Autodesk Inventor part; units mm, degrees
ref_plane "YZ Plane" through (0, 0, 0) normal (1, 0, 0) x (0, 1, 0)
ref_plane "XZ Plane" through (0, 0, 0) normal (0, 1, 0) x (-1, 0, 0)
ref_plane "XY Plane" through (0, 0, 0) normal (0, 0, 1) x (1, 0, 0)
sketch "スケッチ1" plane through (0, 0, 0) normal (0, 0, 1) x (1, 0, 0)
  line L0 (67.5, 17.5) -> (-67.5, 17.5) construction
  line L1 (-67.5, 17.5) -> (-67.5, -17.5) construction
  line L2 (-67.5, -17.5) -> (67.5, -17.5) construction
  line L3 (67.5, -17.5) -> (67.5, 17.5) construction
  line L4 (67.5, 17.5) -> (-67.5, -17.5) construction
  line L5 (-67.5, 17.5) -> (67.5, -17.5) construction
  circle A0 centre (-60, 35) radius 1.6
  circle A1 centre (-70, 35) radius 1.6
  line L6 (-77.5, 27.5) -> (-53, 27.5)
  line L7 (-53, 27.5) -> (-53, 42.5)
  line L8 (-53, 42.5) -> (-80, 42.5) construction
  line L9 (-77.5, 27.5) -> (-77.5, -27.5)
  line L10 (-77.5, -27.5) -> (-50, -27.5)
  circle A2 centre (-60, -35) radius 1.6
  circle A3 centre (-70, -35) radius 1.6
  circle A4 centre (-80, -35) radius 1.6
  line L11 (124.2308, -31.7536) -> (484.5935, -392.1164)
  line L12 (484.5935, -392.1164) -> (488.7129, -553.575)
  line L13 (-80, 21.2868) -> (-468.838, -367.5512) construction
  line L14 (-468.838, -367.5512) -> (-479.4446, -356.9446)
  line L15 (-479.4446, -356.9446) -> (-90.6066, 31.8934) construction
  line L16 (-90.6066, 31.8934) -> (-80, 21.2868) construction
  line L17 (-80, 42.5) -> (-80, 5.3052) construction
  circle A5 centre (-92.3744, 19.519) radius 1.6
  circle A6 centre (-102.981, 8.9124) radius 1.6
  circle A7 centre (-113.5876, -1.6942) radius 1.6
  line L18 (-92.3744, 19.519) -> (-113.5876, -1.6942) construction
  circle A8 centre (-433.75, -321.8566) radius 1.6
  circle A9 centre (-421.9492, -310.0558) radius 1.6
  line L19 (-388.4374, -772.2067) -> (-358.1265, -754.7067) construction
  line L20 (-358.1265, -754.7067) -> (-425.6265, -637.7933) construction
  line L21 (-455.9374, -655.2933) -> (-358.1265, -754.7067) construction
  line L22 (-388.4374, -772.2067) -> (-425.6265, -637.7933) construction
  line L23 (-455.9374, -655.2933) -> (-388.4374, -772.2067) construction
  line L24 (-425.6265, -637.7933) -> (-455.9374, -655.2933) construction
  line L25 (455.9374, -655.2933) -> (425.6265, -637.7933) construction
  line L26 (425.6265, -637.7933) -> (358.1265, -754.7067) construction
  line L27 (388.4374, -772.2067) -> (425.6265, -637.7933) construction
  line L28 (455.9374, -655.2933) -> (358.1265, -754.7067) construction
  line L29 (388.4374, -772.2067) -> (455.9374, -655.2933) construction
  line L30 (358.1265, -754.7067) -> (388.4374, -772.2067) construction
  line L31 (0, 0) -> (0, -263.4473) construction
  line L32 (67.5, 17.5) -> (67.5, -17.5) construction
  circle A10 centre (60, 35) radius 1.6
  circle A11 centre (70, 35) radius 1.6
  line L33 (77.5, 27.5) -> (53, 27.5)
  line L34 (53, 27.5) -> (53, 42.5)
  line L35 (53, 42.5) -> (80, 42.5)
  line L36 (77.5, 27.5) -> (77.5, -27.5)
  line L37 (77.5, -27.5) -> (50, -27.5)
  line L38 (50, -27.5) -> (72.3664, -42.5)
  line L39 (72.3664, -42.5) -> (99.3664, -42.5)
  circle A12 centre (60, -35) radius 1.6
  circle A13 centre (70, -35) radius 1.6
  circle A14 centre (80, -35) radius 1.6
  line L40 (80, 42.5) -> (80, 5.3052) construction
  line L41 (-483.838, -367.5512) -> (-468.838, -367.5512)
  line L42 (-468.838, -367.5512) -> (-468.838, -648.3077)
  line L43 (-468.838, -648.3077) -> (-483.838, -648.3077)
  line L44 (-483.838, -648.3077) -> (-483.838, -367.5512)
  line L45 (-283.2277, -604.4352) -> (-262.2277, -640.8083) construction
  line L46 (345.2492, -497.0108) -> (305.7786, -565.3759) construction
  line L47 (265.1134, -631.6538) -> (-234.8866, -631.6538) construction
  line L48 (-234.8866, -631.6538) -> (-234.8866, -1131.6538) construction
  line L49 (-234.8866, -1131.6538) -> (265.1134, -1131.6538) construction
  line L50 (265.1134, -1131.6538) -> (265.1134, -631.6538) construction
  line L51 (265.1134, -631.6538) -> (-234.8866, -1131.6538) construction
  line L52 (-234.8866, -631.6538) -> (265.1134, -1131.6538) construction
  line L53 (-12.841, -157.5) -> (15.1134, -157.5) construction
  circle A15 centre (1.1362, -409.4569) radius 212.5 construction
  line L54 (501.1362, 53.616) -> (-498.8638, 53.616) construction
  line L55 (-498.8638, 53.616) -> (-498.8638, -946.384) construction
  line L56 (-498.8638, -946.384) -> (501.1362, -946.384) construction
  line L57 (501.1362, -946.384) -> (501.1362, 53.616) construction
  line L58 (501.1362, 53.616) -> (-498.8638, -946.384) construction
  line L59 (-498.8638, 53.616) -> (501.1362, -946.384) construction
  circle A16 centre (1.1362, -409.4569) radius 250 construction
  line L60 (-80, 42.5) -> (-90.6066, 31.8934) construction
  line L61 (-80, 42.5) -> (-118.8909, 3.6091)
  line L62 (-118.8909, -6.9975) -> (-113.5876, -12.3008)
  line L63 (-113.5876, -12.3008) -> (-87.5, -42.5)
  arc A17 (-118.8909, 3.6091) -> (-118.8909, -6.9975) centre (-113.5876, -1.6942) ccw
  line L64 (-80, 42.5) -> (-53, 42.5)
  circle A18 centre (-66, -52.5) radius 1.6
  circle A19 centre (-66, -62.5) radius 1.6
  circle A20 centre (-66, -72.5) radius 1.6
  line L65 (-58.5, -80) -> (-73.5, -80)
  line L66 (-73.5, -80) -> (-87.5, -42.5)
  line L67 (-50, -27.5) -> (-50, -42.5)
  line L68 (-50, -42.5) -> (-58.5, -80)
  point P0 (0, -470)
  point P1 (-102.981, 8.9124)
  point P2 (-77.5, 0)
  point P3 (-407.0319, -705)
  point P4 (-407.0319, -705)
  point P5 (407.0319, -705)
  point P6 (407.0319, -705)
  point P7 (77.5, 0)
  point P8 (15.1134, -881.6538)
  point P9 (1.1362, -446.384)
  point P10 (-124.1942, -1.6942)
  dimension "d27" = 135
  dimension "d28" = 35
  dimension "d29" = 3.2
  dimension "d30" = 3.2
  dimension "d31" = 10
  dimension "d32" = 15
  dimension "d33" = 10
  dimension "d34" = 7.5
  dimension "d35" = 7
  dimension "d36" = 70
  dimension "d37" = 3.2
  dimension "d38" = 3.2
  dimension "d39" = 3.2
  dimension "d40" = 10
  dimension "d41" = 10
  dimension "d45" = 10
  dimension "d46" = 10
  dimension "d53" = 135
  dimension "d54" = 15
  dimension "d55" = 10
  dimension "d57" = 3.2
  dimension "d58" = 3.2
  dimension "d59" = 3.2
  dimension "d60" = 10
  dimension "d61" = 15
  dimension "d62" = 15
  dimension "d63" = 7.5
  dimension "d64" = 45
  dimension "d65" = 3.2
  dimension "d66" = 3.2
  dimension "d69" = 360
  dimension "d76" = 470
  dimension "d77" = 15
  dimension "d80" = 500
  dimension "d81" = 500
  dimension "d82" = 200
  dimension "d83" = 425
  dimension "d84" = 1000
  dimension "d85" = 1000
  dimension "d88" = 42
  dimension "d89" = 500
  dimension "d90" = 7.5
  dimension "d91" = 7.5
  dimension "d112" = 3.2
  dimension "d113" = 3.2
  dimension "d114" = 3.2
  dimension "d115" = 10
  dimension "d116" = 10
  dimension "d117" = 25
  dimension "d118" = 66
  dimension "d120" = 7.5
  dimension "d121" = 7.5
  dimension "d122" = 7.5
  dimension "d123" = 7.5
  dimension "d124" = 7.5
  dimension "d129" = 10
  dimension "d130" = 7.5
  dimension "d131" = 7.5
extrude "押し出し1" add sketch "スケッチ1" along normal blind 3 contours L9 L10 L67 L68 L65 L66 L63 L62 A17 L61 L64 L7 L6
fillet "フィレット1" radius 3 10 edges at (-113.5876, -12.3008, 1.5) (-50, -27.5, 1.5) (-77.5, -27.5, 1.5) (-77.5, 27.5, 1.5) (-53, 27.5, 1.5) (-53, 42.5, 1.5) (-80, 42.5, 1.5) (-87.5, -42.5, 1.5) (-73.5, -80, 1.5) (-58.5, -80, 1.5)
sketch "スケッチ2" plane through (0, 0, 3) normal (0, 0, 1) x (1, 0, 0)
  line L0 (-108.1182, -9.4538) -> (-94.6826, -25.0069)
  line L1 (-83.5, -14.6862) -> (-83.5, 12.9584)
  line L2 (-86.9142, 14.3726) -> (-93.4726, 7.8142)
  line L3 (-77.5, -24.5) -> (-77.5, 24.5)
  line L4 (-80.8787, 41.6213) -> (-118.8909, 3.6091)
  line L5 (-113.516, -12.3836) -> (-87.852, -42.0925)
  line L6 (-96.7234, 4.5634) -> (-83.5, -37.9521) construction
  line L7 (-98.1366, -0.994) -> (-91.2594, -23.1055)
  line L8 (-93.9681, 5.806) -> (-87.4098, -15.2802)
  line L9 (-101.4606, -0.1738) -> (-108.019, -6.7322)
  arc A0 (-98.1366, -0.994) -> (-101.4606, -0.1738) centre (-100.0464, -1.588) ccw
  arc A1 (-93.4726, 7.8142) -> (-93.9681, 5.806) centre (-92.0583, 6.4) ccw
  arc A2 (-94.6826, -25.0069) -> (-91.2594, -23.1055) centre (-93.1692, -23.6995) ccw
  arc A3 (-87.4098, -15.2802) -> (-83.5, -14.6862) centre (-85.5, -14.6862) ccw
  arc A4 (-83.5, 12.9584) -> (-86.9142, 14.3726) centre (-85.5, 12.9584) ccw
  arc A5 (-108.019, -6.7322) -> (-108.1182, -9.4538) centre (-106.6047, -8.1464) ccw
  line L10 (-53, -27.5) -> (-74.5, -27.5)
  point P0 (0, 0)
  point P1 (-99.1198, 2.167)
  dimension "d95" = 6
  dimension "d97" = 15
  dimension "d98" = 6
  dimension "d99" = 3
  dimension "d100" = 3
  dimension "d101" = 2
  dimension "d102" = 2
extrude "押し出し2" cut sketch "スケッチ2" against normal blind 3
properties part number "オムニ_後ろ側板" material "アルミニウム 6061"
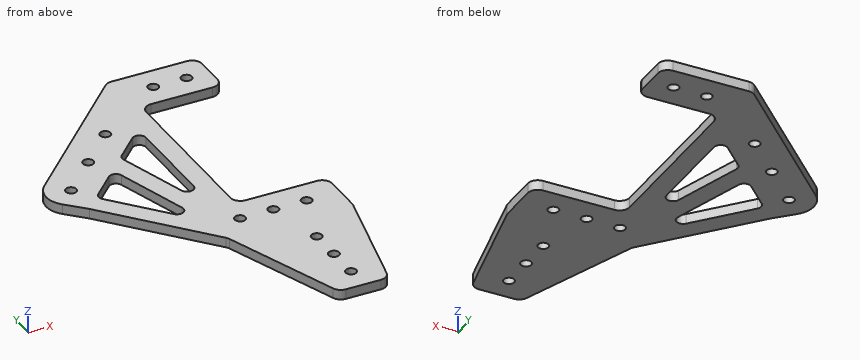
For this review, take the finished solid that the model builds, in its own axes (mm). Round coordinates to 2 decimals unless told otherwise and drop trailing zeros. Order: outer loops, then holes, each group sorted by start corner. A loop starts at its lowest first (then second) coordinate and runs counter-clockwise, first axis right, second up. Notation, with made-up numbers: M 65.5,74 L 100.5,74 A22 ccw 100.5,98 Z; hole C 1,86 d10. An arc over 180 degrees is marked long. Use a Markdown table: item, result. Add a question column.
Item 1: To check wall thickness, follow line 1 along Y through (x, z) = (-66, 1.55); line 2 along Y through (x, z) = (-70, 2.15); line 3 along X through (y, z) = (-12.5, 0.4). State the ranges of each line that lie inside material, in increasing order.
Item 2: Add section B-B, the plane x = -66. Give the boundary of the cut face in (y, z).
Item 3: Add section A-A, the plane y = -72.5. Give the boundary of the cut face in (x, z).
Item 4: Add section D-D, the plane z = 0.8. State how many separate pieces and enclosed holes the cut face has, then the cut area to 3 significant figures.
Item 5: Add section C-C, the plane y = -35. Give the boundary of the cut face in (x, z).
Geometry results:
| question | item | result |
|---|---|---|
| 1 | line 1 | y = -80 to -74.1, -70.9 to -64.1, -60.9 to -54.1, -50.9 to -27.5, 27.5 to 42.5 |
| 1 | line 2 | y = -80 to -36.6, -33.4 to -27.5, 27.5 to 33.4, 36.6 to 42.5 |
| 1 | line 3 | x = -113.42 to -105.49, -94.56 to -88.27, -83.5 to -77.5 |
| 2 | outline | M -80,0 L -74.1,0 L -74.1,3 L -80,3 Z; M -70.9,0 L -64.1,0 L -64.1,3 L -70.9,3 Z; M -60.9,0 L -54.1,0 L -54.1,3 L -60.9,3 Z; M -50.9,0 L -27.5,0 L -27.5,3 L -50.9,3 Z; M 27.5,0 L 42.5,0 L 42.5,3 L 27.5,3 Z |
| 3 | outline | M -76.3,0 L -67.6,0 L -67.6,3 L -76.3,3 Z; M -64.4,0 L -56.8,0 L -56.8,3 L -64.4,3 Z |
| 4 | separate pieces | 1 |
| 4 | enclosed holes | 13 |
| 4 | area | 3,450 mm² |
| 5 | outline | M -93.98,0 L -81.6,0 L -81.6,3 L -93.98,3 Z; M -78.4,0 L -71.6,0 L -71.6,3 L -78.4,3 Z; M -68.4,0 L -61.6,0 L -61.6,3 L -68.4,3 Z; M -58.4,0 L -50,0 L -50,3 L -58.4,3 Z |
